from build123d import *

# Parameters (mm, degrees)
SKETCH1_W           = 72.2
SKETCH1_H           = 44
BOSS_EXTRUDE1_DEPTH = 12.7
BOSS_EXTRUDE2_DEPTH = 12.7
SKETCH1_5_R         = 4.5
SKETCH1_5_R_2       = 1.6
CUT_EXTRUDE3_DEPTH  = 90.878417877
FILLET1_R           = 3.175


with BuildPart() as part:
    # Sketch1 → Boss-Extrude1 (new body)
    with BuildSketch(Plane.XY):
        with Locations((36.1, -22)):
            Rectangle(SKETCH1_W, SKETCH1_H)
    extrude(amount=BOSS_EXTRUDE1_DEPTH)

    # Sketch2 → Boss-Extrude2 (add)
    with BuildSketch(Plane.XY.offset(12.7)):
        Polygon((72.2, -44), (0, -44), (0, 0), (-5, 0), (-5, -52), (72.2, -52), align=None)
    extrude(amount=-BOSS_EXTRUDE2_DEPTH)

    # Sketch1<5> → Cut-Extrude3 (cut, through all)
    with BuildSketch(Plane.XY):
        with Locations((52.5, -22)):
            Circle(SKETCH1_5_R)
        with Locations((7.5, -37)):
            Circle(SKETCH1_5_R_2)
        with Locations((7.5, -7)):
            Circle(SKETCH1_5_R_2)
        with Locations((37.5, -7)):
            Circle(SKETCH1_5_R_2)
        with Locations((37.5, -37)):
            Circle(SKETCH1_5_R_2)
    extrude(amount=CUT_EXTRUDE3_DEPTH, mode=Mode.SUBTRACT)

    # Fillet1
    fillet1_edges = [part.edges().sort_by_distance(p)[0] for p in [
        (72.2, 0, 6.35),
        (-5, 0, 6.35),
        (72.2, -52, 6.35),
        (-5, -52, 6.35),
    ]]
    fillet(fillet1_edges, radius=FILLET1_R)


solid = part.part
Read the model definition and answer for the solid it produces. Units are mm, in the model's axes. Coordinates: 2 decimals unless noted, no trailing zeros. Order: outer loops, then holes, each group sorted by start corner. A loop starts at its lowest first (then second) coordinate and runs counter-clockwise, first axis right, second up. Notation, with made-up numbers: (37, 8) - (47, 8) arc R25 cw to (47, 41) - close; hole circle Ø2 at (43.5, 21). An arc over 180 degrees is marked (long way). Use one line per item in the form item = value.
(1) For a pull along X with two mould halves and no side action, classify faces 1 (the face through (-4.09, -51.05, 6.26)), 2 (the face through (8.24, -38.42, 6.26)), 3 (the face through (72.2, -26, 6)) as pulls with the +X half, pulls with the -X half, needs draft (parallel to the pull), parting line crosses it, or undercut.
Computed values:
face_1 = pulls with the -X half
face_2 = undercut
face_3 = pulls with the +X half
(2) Section B-B, the plane z = 4 is taken. Give the vertices of the cut face in (x, y) (3 decimals), then the cut area to 3 significant figures.
Computed values:
outline = (-5, -48.825) arc R3.175 ccw to (-1.825, -52) - (69.025, -52) arc R3.175 ccw to (72.2, -48.825) - (72.2, -3.175) arc R3.175 ccw to (69.025, 0) - (-1.825, 0) arc R3.175 ccw to (-5, -3.175) - close; hole circle Ø3.2 at (7.5, -37); hole circle Ø3.2 at (7.5, -7); hole circle Ø3.2 at (37.5, -37); hole circle Ø3.2 at (37.5, -7); hole circle Ø9 at (52.5, -22)
area = 3,910 mm²
(3) Section C-C, the plane x = 51 is taken. Give the vertices of the cut face in (y, z), then the cut area to 3 significant figures.
Computed values:
outline = (-52, 0) - (-26.24, 0) - (-26.24, 12.7) - (-52, 12.7) - close; (-17.76, 0) - (0, 0) - (0, 12.7) - (-17.76, 12.7) - close
area = 553 mm²
(4) Straight lines are drawn through the part: L1, parallel to X at y = -7, z = 4.5; L2, parallel to Y at x = 37.5, z = 8.5; L3, parallel to X at y = -36, z = 11.25. For each, find the intervals that lie inside material, in ascending order.
Computed values:
L1 = -5 to 5.9, 9.1 to 35.9, 39.1 to 72.2
L2 = -52 to -38.6, -35.4 to -8.6, -5.4 to 0
L3 = -5 to 6.25, 8.75 to 36.25, 38.75 to 72.2
(5) Section D-D, the plane y = -22 is taken. Give the vertices of the cut face in (x, z).
Computed values:
outline = (-5, 0) - (48, 0) - (48, 12.7) - (-5, 12.7) - close; (57, 0) - (72.2, 0) - (72.2, 12.7) - (57, 12.7) - close
(6) Given pin 1 Ø1.9 at (x, y) = (37.5, -7) entering from +Z, flat-ended and moving along its own axis, determine where the tip first touches the part or whether it passes through.
Computed values:
pin_1 = through
(7) Section A-A, the plane y = -7 is taken. Give the vertices of the cut face in (x, z).
Computed values:
outline = (-5, 0) - (5.9, 0) - (5.9, 12.7) - (-5, 12.7) - close; (9.1, 0) - (35.9, 0) - (35.9, 12.7) - (9.1, 12.7) - close; (39.1, 0) - (72.2, 0) - (72.2, 12.7) - (39.1, 12.7) - close
